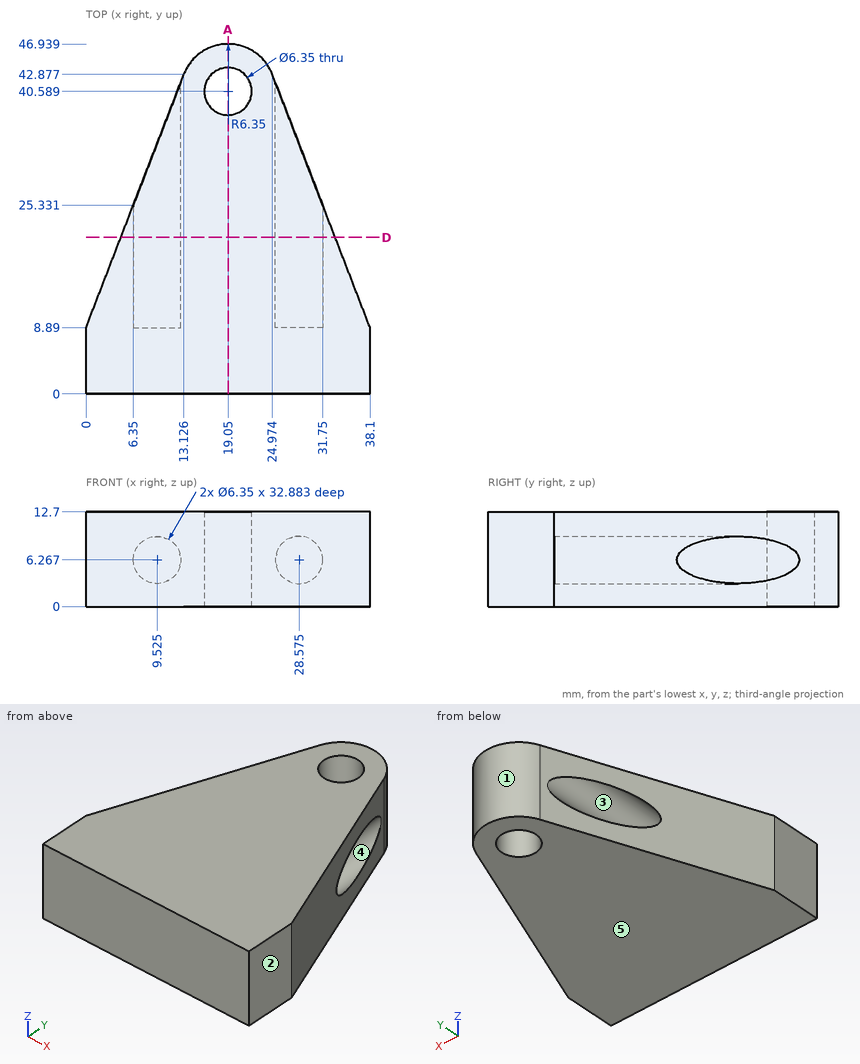
Input: dimensioned drawing with shaded views. Units: mm. Origin: part minimum x, y, z. A direction names the side the tool comes from. Give positions to 0.01 mm unless a question says otherwise; leave off trailing zeros. Loops run counter-clockwise (first coordinate to the right, second up) from the corner with the lowest first, then second, coordinate; pieces in that order, holes last. Notation, with made-up numbers: M 78,35 L 85,35 A29 cw 85,66 Z; hole C 77.5,69.25 d8. An arc over 180 degrees is marked long. Put each result on its own line as item: value.
1) Mould query, pull axis X, two halves, no side actions, for the marked faces 1, 2 and 3. Classes: released by +X, released by -X, zero draft, split by the parting line, or undercut.
Computed values:
face 1: split by the parting line
face 2: released by +X
face 3: undercut
2) Cut plane A-A, the plane x = 19.05. Return the cut outline in (y, z) (1 decimal).
Computed values:
outline: M 0,0 L 37.4,0 L 37.4,12.7 L 0,12.7 Z; M 43.8,0 L 46.9,0 L 46.9,12.7 L 43.8,12.7 Z
3) Material intervals for L1, parallel to X at y = 22, z = 4.5 (1 decimal); L2, parallel to X at y = 16, z = 6 (1 decimal); L3, parallel to Y at x = 19.05, z = 4 (1 decimal), sorted ascending. Write a range as from..to.
Computed values:
L1: x = 5.1..6.9, 12.2..25.9, 31.2..33
L2: x = 2.7..6.4, 12.7..25.4, 31.7..35.4
L3: y = 0..37.4, 43.8..46.9
4) Reachability of the marked faces 4 and 5 from +Z, -Z, +X, -X, +Y, -Y: full face, straight path, thin tool, end or side. Return the list, or none.
Computed values:
face 4: +Y
face 5: -Z, +X, -X, +Y, -Y
5) Cut plane D-D, the plane y = 21. Give the number of separate pieces and of enclosed holes in the cut face, plus the area to 3 significant figures.
Computed values:
separate pieces: 1
enclosed holes: 2
area: 302 mm^2
6) First-contact query: P1, Ø1, axis at y = 35, z = 1.5, coming from the -X side; P2, Ø8, axis at x = 12, y = 23.5, coming from the -Z side; P3, Ø6, axis at y = 35.5, z = 4.5, coming from the -X side; P4, Ø1, axis at y = 41, z = 4, coming from the -X side. Flat tips, straight axial feed; report the tip coordinate or a pass-through.
Computed values:
P1: stops at x = 9.89
P2: stops at z = 0
P3: stops at x = 9.25
P4: stops at x = 12.21
